```python
from build123d import *

# Parameters (mm, degrees)
BOSS_EXTRUDE1_DEPTH      = 3.1
BOSS_EXTRUDE1_DEPTH_BACK = 6
SKETCH1_W                = 41.7
SKETCH1_H                = 74.6
CUT_EXTRUDE1_DEPTH       = 44.151042861
CUT_EXTRUDE1_DEPTH_BACK  = 4
SKETCH2_W                = 37.7
SKETCH2_H                = 65.6
CUT_EXTRUDE2_DEPTH       = 1.75
CUT_EXTRUDE2_DEPTH_BACK  = 0.15
SKETCH3_W                = 36.8
SKETCH3_H                = 2
SKETCH4_W                = 7.7
SKETCH4_H                = 1.7
BOSS_EXTRUDE2_DEPTH      = 4
CUT_EXTRUDE3_START       = 1.6
SKETCH5_R                = 3.1
CUT_EXTRUDE3_DEPTH       = 42.551042861
CUT_EXTRUDE4_DEPTH       = 44.151042861
CUT_EXTRUDE4_DEPTH_BACK  = 5
SKETCH6_R                = 1.05


with BuildPart() as part:
    # Sketch1 → Boss-Extrude1 (new, two sides: drawn at the far end of the back side and taken through both)
    with BuildSketch(Plane(origin=(0, 0, 0), x_dir=(1, 0, 0), z_dir=(0, 1, 0)).offset(-BOSS_EXTRUDE1_DEPTH_BACK)):
        Rectangle(SKETCH1_W, SKETCH1_H)
    extrude(amount=BOSS_EXTRUDE1_DEPTH + BOSS_EXTRUDE1_DEPTH_BACK)

    # Sketch2 → Cut-Extrude1 (cut, two sides: drawn at the far end of the back side and taken through both)
    with BuildSketch(Plane(origin=(0, 0, 0), x_dir=(1, 0, 0), z_dir=(0, 1, 0)).offset(-CUT_EXTRUDE1_DEPTH_BACK)):
        Rectangle(SKETCH2_W, SKETCH2_H)
    extrude(amount=CUT_EXTRUDE1_DEPTH + CUT_EXTRUDE1_DEPTH_BACK, mode=Mode.SUBTRACT)

    # Sketch3 → Cut-Extrude2 (cut, two sides: drawn at the far end of the back side and taken through both)
    with BuildSketch(Plane(origin=(0, 0, 0), x_dir=(1, 0, 0), z_dir=(0, 1, 0)).offset(-CUT_EXTRUDE2_DEPTH_BACK)):
        with Locations((0, -33.8)):
            Rectangle(SKETCH3_W, SKETCH3_H)
    extrude(amount=CUT_EXTRUDE2_DEPTH + CUT_EXTRUDE2_DEPTH_BACK, mode=Mode.SUBTRACT)

    # Sketch4 → Boss-Extrude2 (add)
    with BuildSketch(Plane(origin=(0, 0, 0), x_dir=(1, 0, 0), z_dir=(0, 1, 0))):
        with Locations((-12.4, 31.95)):
            Rectangle(SKETCH4_W, SKETCH4_H)
    extrude(amount=-BOSS_EXTRUDE2_DEPTH)

    # Sketch5 → Cut-Extrude3 (cut, through all)
    with BuildSketch(Plane(origin=(0, 0, 0), x_dir=(1, 0, 0), z_dir=(0, 1, 0)).offset(CUT_EXTRUDE3_START)):
        with Locations((-12.4, 34.05)):
            Circle(SKETCH5_R)
    extrude(amount=CUT_EXTRUDE3_DEPTH, mode=Mode.SUBTRACT)

    # Sketch6 → Cut-Extrude4 (cut, two sides: drawn at the far end of the back side and taken through both)
    with BuildSketch(Plane(origin=(0, 0, 0), x_dir=(1, 0, 0), z_dir=(0, 1, 0)).offset(-CUT_EXTRUDE4_DEPTH_BACK)):
        with Locations(Location((-12.4, 34.05, 0), (0, 0, 270))):
            Circle(SKETCH6_R)
    extrude(amount=CUT_EXTRUDE4_DEPTH + CUT_EXTRUDE4_DEPTH_BACK, mode=Mode.SUBTRACT)


solid = part.part
```
Can you work these out from the model? Positions are in its coordinate system, mm. A direction names the side the tool comes from. Coordinates: 2 decimals unless noted, no trailing zeros. Order: outer loops, then holes, each group sorted by start corner. A loop starts at its lowest first (then second) coordinate and runs counter-clockwise, first axis right, second up. Notation, with made-up numbers: (3.25, -8) - (12.25, -8) arc R20 cw to (12.25, 24) - close; hole circle Ø7 at (55, 76). An arc over 180 degrees is marked (long way). Answer in a Markdown table with one row per item.
1. If I drill on line 1 along Z through (x, y) = (-12.4, -2.75); line 2 along X through (y, z) = (-2.75, -34); line 3 along Z through (x, y) = (-8.5, -2.25), over which ranges is the centre line in solid material (lowest first)?
Reply:
| item | result |
|---|---|
| line 1 | z = -37.3 to -35.1, -33 to -31.1, 32.8 to 37.3 |
| line 2 | x = -20.85 to -13.45, -11.35 to 20.85 |
| line 3 | z = -37.3 to -32.8, 32.8 to 37.3 |
2. Suppose I cut it at C-C (x = 16.5). Please give me the cut outline in (y, z), and give its area (3 significant figures).
Reply:
| item | result |
|---|---|
| outline | (-6, -37.3) - (3.1, -37.3) - (3.1, -32.8) - (-4, -32.8) - (-4, 32.8) - (-0.15, 32.8) - (-0.15, 34.8) - (1.75, 34.8) - (1.75, 32.8) - (3.1, 32.8) - (3.1, 37.3) - (-6, 37.3) - close |
| area | 209 mm^2 |
3. If we mould it in two halves opening along Z, with no side actions, what happens to faces 1 (the flat face through (-20.85, -2, 1)), 2 (the flat face through (18.85, 0, 0)), 3 (the flat face through (0, -2, 37.3))? For each: pulls with the +Z half, pulls with the -Z half, needs draft (parallel to the pull), parting line crosses it, or undercut.
Reply:
| item | result |
|---|---|
| face 1 | needs draft |
| face 2 | undercut |
| face 3 | pulls with the +Z half |
4. For pin 1 (11.5 mm diameter, centred on x = -9, z = -11, fed in from +Y); pin 2 (1.3 mm diameter, centred on x = -13, z = -35, fed in from +Y); pin 3 (1.4 mm diameter, centred on x = -11, z = -32, fed in from +Y), each with a flat end and sliding along its axis, tell me the tip position at first contact or that it passes through.
Reply:
| item | result |
|---|---|
| pin 1 | stops at y = -4 |
| pin 2 | stops at y = 1.6 |
| pin 3 | stops at y = 0 |
5. Suppose I cut it at D-D (z = -34.05). Please give me the cut outline in (x, y).
Reply:
| item | result |
|---|---|
| outline | (-20.85, -6) - (20.85, -6) - (20.85, 3.1) - (-9.3, 3.1) - (-9.3, 1.6) - (-11.35, 1.6) - (-11.35, -5) - (-13.45, -5) - (-13.45, 1.6) - (-15.5, 1.6) - (-15.5, 3.1) - (-20.85, 3.1) - close |
6. For faces 4 (the flat face through (0, -0.15, 34)), 5 (the flat face through (-8.55, -2, -32)), 6 (the flat face through (0, -6, -1)), which set-ups out of +Z, -Z, +X, -X, +Y, -Y let a thin tool reach every point of the face, with its end or its side?
Reply:
| item | result |
|---|---|
| face 4 | none |
| face 5 | +Y |
| face 6 | +Z, -Z, +X, -X, -Y |
7. Suppose I cut it at B-B (z = 6). Please give me the cut outline in (x, y), and give its area (3 significant figures).
Reply:
| item | result |
|---|---|
| outline | (-20.85, -6) - (20.85, -6) - (20.85, 3.1) - (18.85, 3.1) - (18.85, -4) - (-18.85, -4) - (-18.85, 3.1) - (-20.85, 3.1) - close |
| area | 112 mm^2 |
8. Suppose I cut it at A-A (y = -2). Please give me the cut outline in (x, z), and give its area (3 significant figures).
Reply:
| item | result |
|---|---|
| outline | (-20.85, -37.3) - (20.85, -37.3) - (20.85, 37.3) - (-20.85, 37.3) - close; hole (-18.85, -32.8) - (-16.25, -32.8) - (-16.25, -31.1) - (-8.55, -31.1) - (-8.55, -32.8) - (18.85, -32.8) - (18.85, 32.8) - (-18.85, 32.8) - close; hole circle Ø2.1 at (-12.4, -34.05) |
| area | 647 mm^2 |
